```python
from build123d import *

# Parameters (mm, degrees)
SKETCH1_W           = 10.16
SKETCH1_H           = 57.15
SKETCH1_R           = 2.286
BOSS_EXTRUDE1_DEPTH = 22.225
FILLET1_R           = 5.08


with BuildPart() as part:
    # Sketch1 → Boss-Extrude1 (new body)
    with BuildSketch(Plane.XY):
        with Locations((5.08, 28.575)):
            Rectangle(SKETCH1_W, SKETCH1_H)
        with Locations((5.08, 6.35)):
            Circle(SKETCH1_R, mode=Mode.SUBTRACT)
        with Locations((5.08, 25.4)):
            Circle(SKETCH1_R, mode=Mode.SUBTRACT)
        with Locations((5.08, 38.1)):
            Circle(SKETCH1_R, mode=Mode.SUBTRACT)
        with Locations((5.08, 50.8)):
            Circle(SKETCH1_R, mode=Mode.SUBTRACT)
    extrude(amount=BOSS_EXTRUDE1_DEPTH)

    # Fillet1
    fillet1_edges = [part.edges().sort_by_distance(p)[0] for p in [
        (10.16, 0, 11.1125),
        (0, 0, 11.1125),
        (0, 57.15, 11.1125),
        (10.16, 57.15, 11.1125),
    ]]
    fillet(fillet1_edges, radius=FILLET1_R - 0.0001)  # a hair under: the kernel refuses the full size


solid = part.part
```
Input: part model. Units: mm. Frame: model coordinates. Give positions to 0.01 mm unless a question says otherwise; leave off trailing zeros. Order: outer loops, then holes, each group sorted by start corner. A loop starts at its lowest first (then second) coordinate and runs counter-clockwise, first axis right, second up. Notation, with made-up numbers: M 34,-8 L 56,-8 A28 ccw 56,24 Z; hole C 47.25,7.5 d8. An arc over 180 degrees is marked long. Return JSON: item names as keys, results as strings.
1) Section query B-B on z = 6.5. Count the separate pieces of the cut face and the enclosed holes in it, and give its area (3 significant figures).
Taken from the geometry:
{"separate pieces": "1", "enclosed holes": "4", "area": "493 mm2"}
2) Line query: L1, parallel to Y at x = 5.08, z = 10; L2, parallel to X at y = 51, z = 3; L3, parallel to Y at x = 3.25, z = 17. Output: solid intervals per line, ascending. Write a range as [from, to].
Taken from the geometry:
{"L1": "y = [0, 4.06], [8.64, 23.11], [27.69, 35.81], [40.39, 48.51], [53.09, 57.15]", "L2": "x = [0, 2.8], [7.36, 10.16]", "L3": "y = [0.34, 4.98], [7.72, 24.03], [26.77, 36.73], [39.47, 49.43], [52.17, 56.81]"}
3) Section query C-C on x = 1.25. Output: boundary loops of the cut face in (y, z) (3 decimals), and give its area (3 significant figures).
Taken from the geometry:
{"outline": "M 1.743,0 L 55.407,0 L 55.407,22.225 L 1.743,22.225 Z", "area": "1,190 mm2"}
4) Section query A-A on y = 50.8. Output: boundary loops of the cut face in (x, z) (3 decimals).
Taken from the geometry:
{"outline": "M 0,0 L 2.794,0 L 2.794,22.225 L 0,22.225 Z; M 7.366,0 L 10.16,0 L 10.16,22.225 L 7.366,22.225 Z"}
5) Section query D-D on y = 7. Output: boundary loops of the cut face in (x, z) (3 decimals).
Taken from the geometry:
{"outline": "M 0,0 L 2.888,0 L 2.888,22.225 L 0,22.225 Z; M 7.272,0 L 10.16,0 L 10.16,22.225 L 7.272,22.225 Z"}
6) Contact query for flat-ended pins moving along their axis: pin 1 (1.5 mm diameter, centred on x = 8, z = 10, fed in from -Y); pin 2 (5 mm diameter, centred on x = 7.5, z = 6.5, fed in from +Y); pin 3 (4 mm diameter, centred on x = 8.5, z = 11, fed in from +Y); pin 4 (3 mm diameter, centred on x = 8.5, z = 12, fed in from -Y). Output: stop coordinate, or through.
Taken from the geometry:
{"pin 1": "stops at y = 0.49", "pin 2": "stops at y = 57.15", "pin 3": "stops at y = 56.95", "pin 4": "stops at y = 0.38"}
7) Mould query, pull axis Y, two halves, no side actions, for faces 1 (the face through (4.58, 35.87, 10.96)), 2 (the face through (1.449, 55.622, 11.268)), 3 (the face through (4.58, 23.17, 10.96)), 4 (the face through (10.16, 28, 11)). Classes: released by +Y, released by -Y, zero draft, split by the parting line, or undercut.
Taken from the geometry:
{"face 1": "undercut", "face 2": "released by +Y", "face 3": "undercut", "face 4": "zero draft"}
